from build123d import *

# Parameters (mm, degrees)
BOSS_EXTRUDE1_DEPTH                          = 4
CUT_EXTRUDE1_REACH                           = 232.298
SKETCH2_W                                    = 4
SKETCH2_H                                    = 50
CSK_FOR_M4_COUNTERSUNK_FLAT_HEAD_SCR_2_COUNT = 2
CSK_FOR_M4_COUNTERSUNK_FLAT_HEAD_SCR_2_PITCH = 148
CSK_FOR_M4_COUNTERSUNK_FLAT_HEAD_SCR_3_COUNT = 2
CSK_FOR_M4_COUNTERSUNK_FLAT_HEAD_SCR_3_PITCH = 205.104851235
CSK_FOR_M4_COUNTERSUNK_FLAT_HEAD_SCR_4_COUNT = 2
CSK_FOR_M4_COUNTERSUNK_FLAT_HEAD_SCR_4_PITCH = 142


with BuildPart() as part:
    # Sketch1 → Boss-Extrude1 (new body)
    with BuildSketch(Plane.XY):
        Polygon((0, 25), (0, 0), (214, 0), (214, 81), (119, 81), (119, 85), (69, 85), (69, 81), (4, 81), (4, 25), align=None)
        Polygon((0, 0), (0, -25), (4, -25), (4, -81), (69, -81), (69, -85), (119, -85), (119, -81), (214, -81), (214, 0), align=None)
    extrude(amount=BOSS_EXTRUDE1_DEPTH)

    # Sketch2 → Cut-Extrude1 (cut, up to next)
    with BuildSketch(Plane.XY.offset(4), mode=Mode.PRIVATE) as cut_extrude1_sk1:
        with Locations((174, 0)):
            Rectangle(SKETCH2_W, SKETCH2_H)
    cut_extrude1_tool1 = extrude(cut_extrude1_sk1.sketch, amount=-CUT_EXTRUDE1_REACH, mode=Mode.PRIVATE) & part.part
    add(cut_extrude1_tool1.solids().sort_by_distance((174, 0, 4))[0], mode=Mode.SUBTRACT)

    # Sketch4 → CSK for M4 Countersunk Flat Head Screw1 (revolve, cut)
    with BuildSketch(Plane(origin=(14, 71, 4), x_dir=(0, -1, 0), z_dir=(1, 0, 0))):
        Polygon((0, 0), (0, 4), (2.25, 4), (2.25, 2.45), (4.7, 0), align=None)
    csk_for_m4_countersunk_flat_head_screw1 = revolve(axis=Axis((14, 71, 10.35), (0, 0, -1)), mode=Mode.SUBTRACT)

    # CSK for M4 Countersunk Flat Head Scr 2: CSK for M4 Countersunk Flat Head Screw1 ×2
    with Locations(*[(i * CSK_FOR_M4_COUNTERSUNK_FLAT_HEAD_SCR_2_PITCH, 0, 0) for i in range(1, CSK_FOR_M4_COUNTERSUNK_FLAT_HEAD_SCR_2_COUNT)]):
        add(csk_for_m4_countersunk_flat_head_screw1, mode=Mode.SUBTRACT)

    # CSK for M4 Countersunk Flat Head Scr 3: CSK for M4 Countersunk Flat Head Screw1 ×2
    with Locations(*[Vector(0.7215821522946791, -0.6923288217962462, 0) * (i * CSK_FOR_M4_COUNTERSUNK_FLAT_HEAD_SCR_3_PITCH) for i in range(1, CSK_FOR_M4_COUNTERSUNK_FLAT_HEAD_SCR_3_COUNT)]):
        add(csk_for_m4_countersunk_flat_head_screw1, mode=Mode.SUBTRACT)

    # CSK for M4 Countersunk Flat Head Scr 4: CSK for M4 Countersunk Flat Head Screw1 ×2
    with Locations(*[(0, -i * CSK_FOR_M4_COUNTERSUNK_FLAT_HEAD_SCR_4_PITCH, 0) for i in range(1, CSK_FOR_M4_COUNTERSUNK_FLAT_HEAD_SCR_4_COUNT)]):
        add(csk_for_m4_countersunk_flat_head_screw1, mode=Mode.SUBTRACT)


solid = part.part
Input: part model. Units: mm. Frame: model coordinates. Round coordinates to 2 decimals unless told otherwise and drop trailing zeros. Write each loop counter-clockwise with the first axis right and the second up, starting at its lowest first coordinate (ties: lowest second). Pieces come first, ordered by that corner, then holes.
1) Cut plane B-B (x = 162). Return the cut outline in (y, z).
2) Ray query, L1, parallel to X at y = -71, z = 0.6; L2, parallel to Y at x = 14, z = 1.2; L3, parallel to Y at x = 173, z = 1.55. Return the intervals inside material, ascending.
3) Cut plane A-A (y = 19). Return the cut outline in (x, z), then the cut area to 3 significant figures.
4) Cut plane C-C (y = 71). Return the cut outline in (x, z), then the cut area to 3 significant figures.
5) Cut plane D-D (z = 3). Return the cut outline in (x, y), then the cut area to 3 significant figures.
6) Contact query for flat-ended pins moving along their axis: P1, Ø1.2, axis at x = 49.5, z = 3, coming from the +Y side; P2, Ø1.2, axis at x = 173.5, z = 1, coming from the -Y side; P3, Ø1.2, axis at y = 83, z = 2, coming from the +X side. Output: stop coordinate, or through.
7) Draft query along X for faces 1 (the cylindrical face through (160.103, -72.21, 0.786)), 2 (the flat face through (106, 1, 4)), 3 (the cylindrical face through (14.86, -73.08, 0.79)). Return one class per face: pulls with the +X half, pulls with the -X half, needs draft (parallel to the pull), parting line crosses it, or undercut.
Geometry says:
1. outline: (-81, 0) - (-73.25, 0) - (-73.25, 1.55) - (-75.7, 4) - (-81, 4) - close; (-68.75, 0) - (68.75, 0) - (68.75, 1.55) - (66.3, 4) - (-66.3, 4) - (-68.75, 1.55) - close; (73.25, 0) - (81, 0) - (81, 4) - (75.7, 4) - (73.25, 1.55) - close
2. L1: x = 4 to 11.75, 16.25 to 159.75, 164.25 to 214
2. L2: y = -81 to -73.25, -68.75 to 68.75, 73.25 to 81
2. L3: y = -81 to -25, 25 to 81
3. outline: (0, 0) - (172, 0) - (172, 4) - (0, 4) - close; (176, 0) - (214, 0) - (214, 4) - (176, 4) - close
3. area: 840 mm2
4. outline: (4, 0) - (11.75, 0) - (11.75, 1.55) - (9.3, 4) - (4, 4) - close; (16.25, 0) - (159.75, 0) - (159.75, 1.55) - (157.3, 4) - (18.7, 4) - (16.25, 1.55) - close; (164.25, 0) - (214, 0) - (214, 4) - (166.7, 4) - (164.25, 1.55) - close
4. area: 792 mm2
5. outline: (0, -25) - (4, -25) - (4, -81) - (69, -81) - (69, -85) - (119, -85) - (119, -81) - (214, -81) - (214, 81) - (119, 81) - (119, 85) - (69, 85) - (69, 81) - (4, 81) - (4, 25) - (0, 25) - close; hole circle Ø7.4 at (14, -71); hole circle Ø7.4 at (14, 71); hole circle Ø7.4 at (162, -71); hole circle Ø7.4 at (162, 71); hole (172, -25) - (176, -25) - (176, 25) - (172, 25) - close
5. area: 34,200 mm2
6. P1: stops at y = 81
6. P2: stops at y = -81
6. P3: stops at x = 119
7. face 1: undercut
7. face 2: needs draft
7. face 3: undercut
